from build123d import *

# Parameters (mm, degrees)
F0_W      = 139.7
F0_H      = 139.7
F2_DEPTH  = 69.85
F3_W      = 44.45
F3_H      = 50.8
F4_DEPTH  = 101.6
F3_H_2    = 50.8314919436
F6_DEPTH  = 101.6
F8_T      = -2.54
F10_D     = 7.0104
F10_DEPTH = 62.5339166651
F11_D     = 7.0104
F13_DEPTH = 21.0058
F15_DEPTH = 21.0058


with BuildPart() as f2:
    # F0 (on Front) → F2 (new body, symmetric)
    with BuildSketch(Plane.XZ):
        with Locations((7.3170833349, 137.3853212178)):
            Rectangle(F0_W, F0_H)
    extrude(amount=F2_DEPTH, both=True)


with BuildPart() as f4:
    # F3 (on Top) → F4 (new body, symmetric)
    with BuildSketch(Plane.XY):
        with Locations((-34.519743681, 37.2602967441)):
            Rectangle(F3_W, F3_H)
    extrude(amount=F4_DEPTH, both=True)


with BuildPart() as f4b:
    # F3 (on Top) → F4, piece 2 (new body, symmetric)
    with BuildSketch(Plane.XY):
        with Locations((48.030256319, 37.2760427159)):
            Rectangle(F3_W, F3_H_2)
    extrude(amount=F4_DEPTH, both=True)


with BuildPart() as f6:
    # F5 (on Right) → F6 (new body, symmetric)
    with BuildSketch(Plane.YZ):
        Polygon((76.787297499, 66.9550536128), (134.3187632341, 208.0787243784), (-53.84613112, 284.7873453586), (-111.3775968552, 143.663674593), align=None)
    extrude(amount=F6_DEPTH, both=True)


with BuildPart() as f2_1:
    add(f2.part)

    # F7: cut F6
    add(f6.part, mode=Mode.SUBTRACT)

    # F8
    f8_openings = [f2_1.faces().sort_by_distance(p)[0] for p in [
        (7.317083, 0, 98.258702),
    ]]
    offset(amount=F8_T, openings=f8_openings)

    # F9: cut F4b, F4
    add(f4b.part, mode=Mode.SUBTRACT)
    add(f4.part, mode=Mode.SUBTRACT)

    # F10 (through all, one way)
    with BuildSketch(Plane.YZ):
        with Locations((-60.4358874261, 76.2015281631)):
            Circle(F10_D / 2)
    extrude(amount=-F10_DEPTH, mode=Mode.SUBTRACT)

    # F11 (through all)
    with Locations(Plane(origin=(0, 0, 0), x_dir=(0, 1, 0), z_dir=(-1, 0, 0))):
        with Locations((-60.4358874261, -76.2015281631)):
            Hole(F11_D / 2)

    # F12 (on face) → F13 (join)
    with BuildSketch(Plane(origin=(74.6270833349, 0, 0), x_dir=(0, -1, 0), z_dir=(-1, 0, 0))):
        with BuildLine():
            Line((4.7972360938, 82.5531459689), (-5.0022536889, 82.5531459689))
            ThreePointArc((-5.0022536889, 82.5531459689), (-8.2025087976, 76.1031459689), (-5.0022536889, 69.6531459689))
            Line((-5.0022536889, 69.6531459689), (4.8260011356, 69.6750988441))
            ThreePointArc((4.8260011356, 69.6750988441), (7.9974709963, 76.1212384837), (4.7972360938, 82.5531459689))
        make_face()
    extrude(amount=F13_DEPTH)

    # F14 (on face) → F15 (join)
    with BuildSketch(Plane.YZ.offset(-59.9929166651)):
        with BuildLine():
            Line((4.7729444071, 82.9956434011), (-5.0265453756, 82.9956434011))
            ThreePointArc((-5.0265453756, 82.9956434011), (-8.2268004843, 76.5456434011), (-5.0265453756, 70.0956434011))
            Line((-5.0265453756, 70.0956434011), (4.8017094489, 70.1175962763))
            ThreePointArc((4.8017094489, 70.1175962763), (7.9731793096, 76.5637359159), (4.7729444071, 82.9956434011))
        make_face()
    extrude(amount=F15_DEPTH)


solid = f2_1.part
Can you work these out from the model? Positions are in its coordinate system, mm. A direction names the side the tool comes from. Give positions to 0.01 mm unless a question says otherwise; leave off trailing zeros. Loops run counter-clockwise (first coordinate to the right, second up) from the corner with the lowest first, then second, coordinate; pieces in that order, holes last. Notation, with made-up numbers: (25, 51) -> (69, 51) arc R22 ccw to (69, 59) -> close; hole circle Ø2 at (34.25, -5). An arc over 180 degrees is marked (long way). Use one line per item in the form item = value.
1) If we section it at B-B (x = -43): Please give me the cut outline in (y, z), plus the area to 3 significant figures.
Answers:
outline = (-69.85, 67.54) -> (11.86, 67.54) -> (11.86, 70.08) -> (-67.31, 70.08) -> (-67.31, 125.7) -> (-69.85, 126.73) -> close; (-5.03, 70.1) -> (4.8, 70.12) arc R8.1 ccw to (4.77, 83) -> (-5.03, 83) arc R8.1 ccw to start; (62.66, 67.54) -> (69.85, 67.54) -> (69.85, 69.78) -> (67.31, 70.82) -> (67.31, 70.08) -> (62.66, 70.08) -> close
area = 553 mm²
2) If we section it at D-D (z = 112.5): Please give me the cut outline in (x, y), plus the area to 3 significant figures.
Answers:
outline = (-62.53, -69.85) -> (77.17, -69.85) -> (77.17, -34.93) -> (74.63, -34.93) -> (74.63, -67.31) -> (-59.99, -67.31) -> (-59.99, -34.93) -> (-62.53, -34.93) -> close
area = 519 mm²
3) Will these pins go through, and if not, where does the flat tip stop? pin 1 (5 mm diameter, centred on x = 62, y = -2, fed in from +Z); pin 2 (5 mm diameter, centred on x = 26, y = 13.5, fed in from +Z); pin 3 (3 mm diameter, centred on x = -22.5, z = 118.5, fed in from +Y).
Answers:
pin_1 = 82.55
pin_2 = 70.08
pin_3 = -67.31
4) If we section it at C-C (y = 47): Please give me the cut outline in (x, z).
Answers:
outline = (-62.53, 67.54) -> (-56.74, 67.54) -> (-56.74, 70.08) -> (-59.99, 70.08) -> (-59.99, 79.1) -> (-62.53, 79.1) -> close; (-12.29, 67.54) -> (25.81, 67.54) -> (25.81, 70.08) -> (-12.29, 70.08) -> close; (70.26, 67.54) -> (77.17, 67.54) -> (77.17, 79.1) -> (74.63, 79.1) -> (74.63, 70.08) -> (70.26, 70.08) -> close
5) I need wall thicknesses on line 1 along X through (y, z) = (-41, 114); line 2 along Z through (x, y) = (71.5, -36); line 3 along Y through (x, z) = (52, 116). Which ranges of each line are inside material? Lowest first, please.
Answers:
line_1 = -62.53 to -59.99, 74.63 to 77.17
line_2 = 67.54 to 70.08
line_3 = -69.85 to -67.31
6) If we section it at A-A (x = 35.5): Please give me the cut outline in (y, z), plus the area to 3 significant figures.
Answers:
outline = (-69.85, 67.54) -> (11.86, 67.54) -> (11.86, 70.08) -> (-67.31, 70.08) -> (-67.31, 125.7) -> (-69.85, 126.73) -> close; (62.69, 67.54) -> (69.85, 67.54) -> (69.85, 69.78) -> (67.31, 70.82) -> (67.31, 70.08) -> (62.69, 70.08) -> close
area = 369 mm²
7) We'd pull the mould along Y, two halves only. Please class faces 3 (the face through (74.906, -31.37, 111.047)), 4 (the face through (-49.637, -8.226, 76.65)), 5 (the face through (-50, 0, 82.996)): released by +Y, released by -Y, zero draft, split by the parting line, or undercut.
Answers:
face_3 = released by +Y
face_4 = undercut
face_5 = zero draft
8) For faces 1 (the face through (-62.533, -17, 90)), 2 (the face through (64.271, -7.994, 76.335)), which set-ups out of +Z, -Z, +X, -X, +Y, -Y let a thin tool reach every point of the face, with its end or its side?
Answers:
face_1 = +Z, -Z, -X, +Y, -Y
face_2 = none
